from build123d import *

# Parameters (mm, degrees)
BOSS_EXTRUDE1_DEPTH = 6.35
SKETCH3_R           = 1
CUT_EXTRUDE3_DEPTH  = 10


with BuildPart() as part:
    # Sketch1 → Boss-Extrude1 (new body)
    with BuildSketch(Plane.XY):
        Polygon((0, 0), (1.5875, 0), (1.5875, 2.38125), (4.7625, 2.38125), (4.7625, 0), (6.35, 0), (6.35, 812.8), (4.7625, 812.8), (4.7625, 800.1), (1.5875, 800.1), (1.5875, 812.8), (0, 812.8), align=None)
    extrude(amount=BOSS_EXTRUDE1_DEPTH)

    # Sketch3 → Cut-Extrude3 (cut, symmetric)
    with BuildSketch(Plane(origin=(0, 0, 0), x_dir=(0, 0, -1), z_dir=(1, 0, 0))):
        with Locations((-3.175, 806.45)):
            Circle(SKETCH3_R)
    extrude(amount=CUT_EXTRUDE3_DEPTH, both=True, mode=Mode.SUBTRACT)


solid = part.part
Work out the finished part from the listing and answer in its coordinate system (mm). Round coordinates to 2 decimals unless told otherwise and drop trailing zeros. Loops run counter-clockwise (first coordinate to the right, second up) from the corner with the lowest first, then second, coordinate; pieces in that order, holes last. Notation, with made-up numbers: M -40,-3 L 12,-3 A14 cw 12,4 Z; hole C 6.25,60 d2. An arc over 180 degrees is marked long. One line per question, with ' | ' between items. Start each with the question number.
(1) Find the intervals of material crossed by line 1 (Z direction, x = 5.6, y = 806.45) (3 decimals); line 2 (Y direction, x = 2.5, z = 3.5), in increasing order.
(2) A cutting plane is placed at A-A on x = 3.5. Write down the section's boundary in (y, z).
(3) Flat-ended cylindrical pins translate along their axes: pin 1 Ø1 at (x, z) = (3.5, 3.5) entering from -Y; pin 2 Ø1.6 at (y, z) = (806.45, 3.175) entering from -X; pin 3 Ø1.5 at (x, z) = (3.5, 2) entering from +Y. Find the tip coordinate at first contact, or state that the pin passes through.
Geometry check:
1) line 1: z = 0 to 2.175, 4.175 to 6.35 | line 2: y = 2.38 to 800.1
2) outline: M 2.38,0 L 800.1,0 L 800.1,6.35 L 2.38,6.35 Z
3) pin 1: stops at y = 2.38 | pin 2: passes through | pin 3: stops at y = 800.1
